Answer from the drawing. Dimensions are ordinates in mm from the lowest x, y and z of the part. A direction names the side the tool comes from. Give positions to 0.01 mm unless a question says otherwise; leave off trailing zeros. Write each loop counter-clockwise with the first axis right and the second up, starting at its lowest first coordinate (ties: lowest second). Pieces come first, ordered by that corner, then holes. Notation, with made-up numbers: M 25.25,57.25 L 32.25,57.25 A23 cw 32.25,71.25 Z; hole C 53,87.5 d7. An arc over 180 degrees is marked long. Write each question's results on one line, items separated by ' | '. Start each with the question number.
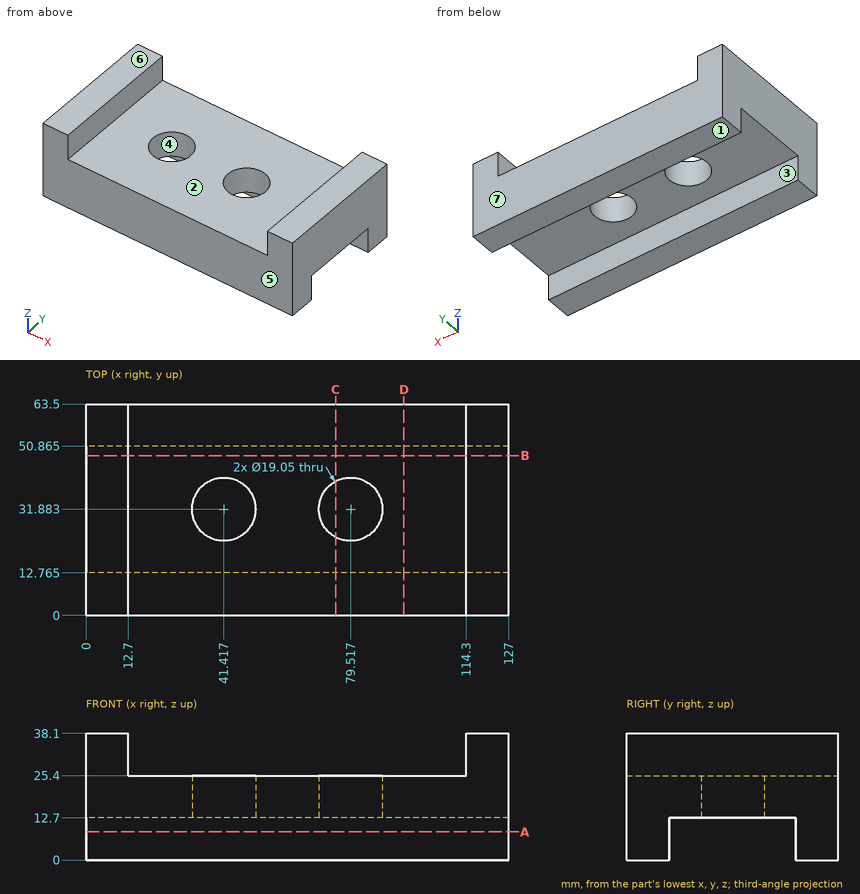
Item 1: Section A-A, the plane z = 8.5 is taken. Determine the outline of the cut face in (x, y) (1 decimal).
Item 2: For the marked faces 1, 2 and 3, determine the directions among +Z, -Z, +X, -X, +Y, -Y from which every point of the face is accessible in a straight line to the end or side of a thin tool.
Item 3: Section D-D, the plane x = 95.5 is taken. Determine the outline of the cut face in (y, z) (1 decimal).
Item 4: Determine the mould class of the marked faces 4, 5, 6 and 7 for opening direction Y: +Y half, -Y half, draft (parallel to the pull), parting line (faces both ways), or undercut.
Item 5: Section B-B, the plane y = 48 is taken. Determine the outline of the cut face in (x, z).
Item 6: Section C-C, the plane x = 75 is taken. Determine the outline of the cut face in (y, z) (1 decimal), then the cut area to 3 significant figures.
Item 7: Given P1, Ø25, axis at x = 41.42, y = 31.88, coming from the +Z side; P2, Ø17, axis at x = 79.52, y = 31.88, coming from the +Z side; P3, Ø10, axis at x = 71, z = 20.5, coming from the -Y side, each flat-ended and moving along its own axis, determine where each tip first touches the part or whether it passes through.
Item 8: Straight lines are drawn through the part: line 1 (X direction, y = 32, z = 22); line 2 (Y direction, x = 31.5, z = 11) (1 decimal); line 3 (X direction, y = 10, z = 26). For each, find the intervals that lie inside material, in ascending order.
Worked out:
1) outline: M 0,0 L 127,0 L 127,12.8 L 0,12.8 Z; M 0,50.9 L 127,50.9 L 127,63.5 L 0,63.5 Z
2) face 1: -Z, +X, -X, +Y, -Y | face 2: +Z, +Y, -Y | face 3: -Z, +X, -X
3) outline: M 0,0 L 12.8,0 L 12.8,12.7 L 50.9,12.7 L 50.9,0 L 63.5,0 L 63.5,25.4 L 0,25.4 Z
4) face 4: undercut | face 5: -Y half | face 6: draft | face 7: +Y half
5) outline: M 0,12.7 L 127,12.7 L 127,38.1 L 114.3,38.1 L 114.3,25.4 L 12.7,25.4 L 12.7,38.1 L 0,38.1 Z
6) outline: M 0,0 L 12.8,0 L 12.8,12.7 L 23.5,12.7 L 23.5,25.4 L 0,25.4 Z; M 40.3,12.7 L 50.9,12.7 L 50.9,0 L 63.5,0 L 63.5,25.4 L 40.3,25.4 Z | area: 916 mm²
7) P1: stops at z = 25.4 | P2: passes through | P3: stops at y = 0
8) line 1: x = 0 to 31.89, 50.94 to 69.99, 89.04 to 127 | line 2: y = 0 to 12.8, 50.9 to 63.5 | line 3: x = 0 to 12.7, 114.3 to 127
